```python
from build123d import *

# Parameters (mm, degrees)
F0_R     = 10
F0_R_2   = 7.5
F1_DEPTH = 985
F3_DEPTH = 1005


with BuildPart() as f1:
    # F0 (on Top) → F1 (new body)
    with BuildSketch(Plane.XY):
        Circle(F0_R)
        Circle(F0_R_2, mode=Mode.SUBTRACT)
    extrude(amount=F1_DEPTH)


with BuildPart() as f3:
    # F0 (on Top) → F3 (new body)
    with BuildSketch(Plane.XY):
        with Locations((149.209142, -44.897571)):
            Circle(F0_R)
        with Locations((149.209142, -44.897571)):
            Circle(F0_R_2, mode=Mode.SUBTRACT)
    extrude(amount=F3_DEPTH)


solid = f1.part
```
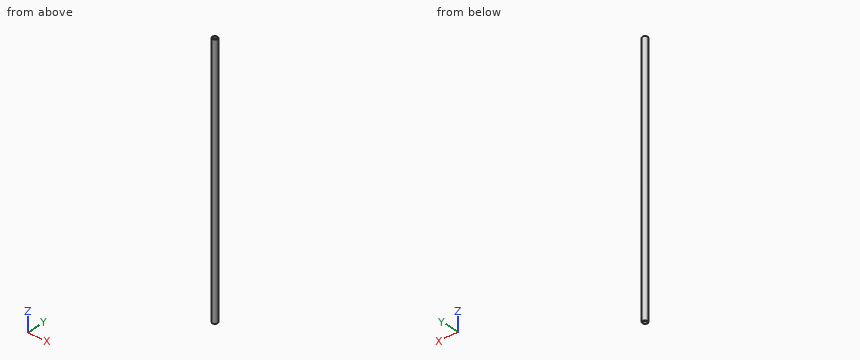
Work out the finished part from the listing and answer in its coordinate system (mm). Coordinates: 2 decimals unless noted, no trailing zeros. Loops run counter-clockwise (first coordinate to the right, second up) from the corner with the lowest first, then second, coordinate; pieces in that order, holes last.
1) Section A-A (x = 0) is taken. Give the vertices of the cut face in (y, z).
Results:
outline: (-10, 0) - (-7.5, 0) - (-7.5, 985) - (-10, 985) - close; (7.5, 0) - (10, 0) - (10, 985) - (7.5, 985) - close
2) Flat-ended cylindrical pins translate along their axes: pin 1 (4 mm diameter, centred on x = 3, z = 791, fed in from -Y); pin 2 (8 mm diameter, centred on y = 0.5, z = 869.5, fed in from -X); pin 3 (4 mm diameter, centred on x = 5.5, z = 726.5, fed in from +Y); pin 4 (3 mm diameter, centred on y = -5.5, z = 459, fed in from -X). Find the tip coordinate at first contact, or state that the pin passes through.
Results:
pin 1: stops at y = -9.95
pin 2: stops at x = -10
pin 3: stops at y = 9.37
pin 4: stops at x = -9.17
3) Consider probe 1 along Y at (x, z) = (-1.25, 165.5); probe 2 along Y at (x, z) = (0, 221); probe 3 along X at (y, z) = (-0.5, 775). Determine where each line is inside the solid, lowest interval first.
Results:
probe 1: y = -9.92 to -7.4, 7.4 to 9.92
probe 2: y = -10 to -7.5, 7.5 to 10
probe 3: x = -9.99 to -7.48, 7.48 to 9.99
4) Section C-C (z = 800) is taken. Give the vertices of the cut face in (x, y), plus the area to 3 significant figures.
Results:
outline: circle Ø20 at (0, 0); hole circle Ø15 at (0, 0)
area: 137 mm2
